Source: CAD feature listing. Evaluate the final solid. Frame: model axes, mm. Face numbers are marked on the shaded views. A direction names the side the tool comes from. Give positions to 0.01 mm unless a question says otherwise; leave off trailing zeros. Loops run counter-clockwise (first coordinate to the right, second up) from the corner with the lowest first, then second, coordinate; pieces in that order, holes last. Notation, with made-up numbers: M 60.5,61 L 103.5,61 A8 ccw 103.5,65 Z; hole C -35,-23 d3. An arc over 180 degrees is marked long. Answer in a Markdown table with one row per item.
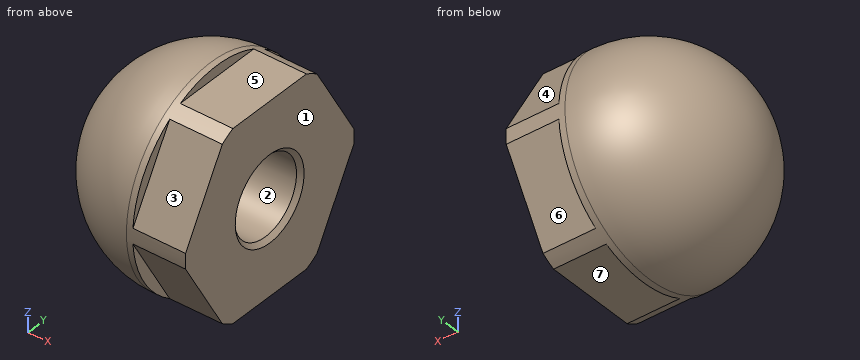
Autodesk Inventor part; units mm, degrees
ref_plane "YZ Plane" through (0, 0, 0) normal (1, 0, 0) x (0, 1, 0)
ref_plane "XZ Plane" through (0, 0, 0) normal (0, 1, 0) x (-1, 0, 0)
ref_plane "XY Plane" through (0, 0, 0) normal (0, 0, 1) x (1, 0, 0)
sketch "Esboço1" plane through (0, 0, 0) normal (0, 0, 1) x (1, 0, 0)
  line L0 (0, 0) -> (-78, 0)
  arc A0 (-28, 50) -> (-78, 0) centre (-28, 0) ccw
  line L1 (-28, 50) -> (0, 50)
  line L2 (0, 50) -> (0, 0)
  line L3 (-106.0264, 0) -> (17.6711, 0)
  dimension "d0" = 28
  dimension "d1" = 50
  dimension "d2" = 50
revolve "Revolução1" add sketch "Esboço1" angle 360 about axis through (-10, 0, 0) along (1, 0, 0)
sketch "Esboço2" plane through (0, 0, 0) normal (1, 0, 0) x (0, 0, -1)
  point P0 (0, 0)
  point P1 (0, 0)
hole "Furo1" at (0, 0, 0) direction (-1, 0, 0) diameter 36.835 depth 50 tip angle 118
chamfer "Chanfro1" distance 2 angle 45 1 edges at (0, 0, 18.4175)
sketch "Esboço3" plane through (0, 0, 0) normal (1, 0, 0) x (0, 0, -1)
  circle A0 centre (0, 0) radius 50
  circle A1 centre (0, 0) radius 20.4175
  line L0 (45, 21.7945) -> (45, -21.7945)
  arc A2 (45, -21.7945) -> (45, 21.7945) centre (0, 0) ccw
  dimension "d14" = 45
extrude "Extrusão1" cut sketch "Esboço3" against normal blind 25 contours A0 L0 picked at (45.9189, -4.9362)
pattern_circular "Padrão circular1" count 6 over 360 about axis through (-10, 0, 0) along (1, 0, 0) of "Extrusão1"
1) Section B-B, the plane z = -30. Return loops of the section in (x, y).
Reply:
| item | result |
|---|---|
| outline | M -28,-40 L -25,-40 L -25,-34.64 L 0,-34.64 L 0,34.64 L -25,34.64 L -25,40 L -28,40 A40 ccw Z |
2) Pull-direction query (Z, two-part tool) for the marked faces 1, 2 and 3; classes: released by +Z, released by -Z, zero draft, split by the parting line, or undercut.
Reply:
| item | result |
|---|---|
| face 1 | zero draft |
| face 2 | undercut |
| face 3 | released by +Z |
3) Pin query (flat end, axial travel): pin 1 Ø20 at (x, y) = (-13.5, 9) entering from +Z; pin 2 Ø2 at (y, z) = (13, 8.5) entering from +X; pin 3 Ø1 at (x, z) = (-69, -8.5) entering from +Y. Return the tip coordinate at first contact, or that it passes through.
Reply:
| item | result |
|---|---|
| pin 1 | stops at z = 45 |
| pin 2 | stops at x = -51.13 |
| pin 3 | stops at y = 28.08 |
4) Section D-D, the plane x = -45. Return loops of the section in (y, z) (1 decimal).
Reply:
| item | result |
|---|---|
| outline | C 0,0 d94; hole C 0,0 d36.8 |
5) Set-up query: the marked faces 4, 5, 6 and 7. Return all of +Z, -Z, +X, -X, +Y, -Y with unobstructed straight access to the full face (end or side cutting, diameter ignored); none if empty.
Reply:
| item | result |
|---|---|
| face 4 | +Z, +X, +Y |
| face 5 | +Z, +X, +Y, -Y |
| face 6 | -Z, +X, +Y |
| face 7 | -Z, +X, +Y, -Y |
6) Material intervals for L1, parallel to Z at x = -15.5, y = 0; L2, parallel to Z at x = -40, y = 0; L3, parallel to X at y = 41, z = 23, sorted ascending.
Reply:
| item | result |
|---|---|
| L1 | z = -45 to -18.42, 18.42 to 45 |
| L2 | z = -48.54 to -18.42, 18.42 to 48.54 |
| L3 | x = -45.03 to -25 |
7) Section A-A, the plane x = -12. Return loops of the section in (y, z) (1 decimal), then the cut area to 3 significant figures.
Reply:
| item | result |
|---|---|
| outline | M -49.9,-3.6 L -28.1,-41.4 A50 ccw -21.8,-45 L 21.8,-45 A50 ccw 28.1,-41.4 L 49.9,-3.6 A50 ccw 49.9,3.6 L 28.1,41.4 A50 ccw 21.8,45 L -21.8,45 A50 ccw -28.1,41.4 L -49.9,3.6 A50 ccw Z; hole C 0,0 d36.8 |
| area | 5,910 mm² |
8) Section C-C, the plane y = 24.5. Return loops of the section in (x, z), then the cut area to 3 significant figures.
Reply:
| item | result |
|---|---|
| outline | M -28,-43.59 L 0,-43.59 L 0,43.59 L -28,43.59 A43.59 ccw Z |
| area | 5,420 mm² |
